Read the model definition and answer for the solid it produces. Units are mm, in the model's axes. A direction names the side the tool comes from. Round coordinates to 2 decimals unless told otherwise and drop trailing zeros. Order: outer loops, then holes, each group sorted by start corner. A loop starts at its lowest first (then second) coordinate and runs counter-clockwise, first axis right, second up. Notation, with made-up numbers: (-15.5, 70) - (-7.5, 70) arc R23 ccw to (-7.5, 86) - close; hole circle Ø9 at (-38, -32.5). An arc over 180 degrees is marked (long way). One line per question, with ' | ' between items. Start each with the question number.
1) For faces 1 (the flat face through (166, -2.794, 38)), 2 (the flat face through (-151, 2.794, -14)), 3 (the flat face through (-151, -2.794, -14)), determine the directions among +Z, -Z, +X, -X, +Y, -Y from which every point of the face is accessible in a straight line to the end or side of a thin tool.
2) The mould has two halves that part along X. Classify faces 4 (the flat face through (157.48, 6, 39)), 5 (the flat face through (166, 2.794, 38)), 6 (the cylindrical face through (-119.669, -0.133, -89.713)): pulls with the +X half, pulls with the -X half, needs draft (parallel to the pull), parting line crosses it, or undercut.
3) Flat-ended cylindrical pins translate along their axes: pin 1 (14 mm diameter, centred on x = -152, z = -16, fed in from -Y); pin 2 (2 mm diameter, centred on x = 55.88, y = 0, fed in from -Z); pin 3 (1 mm diameter, centred on y = 5.5, z = -12, fed in from +X). Find the tip coordinate at first contact, or state that the pin passes through.
4) The part is cut by section B-B, the plane z = -38.1. Give the vertices of the cut face in (x, y) (3 decimals), plus the area to 3 significant figures.
5) The part is cut by section C-C, the plane z = -77.5. Give the vertices of the cut face in (x, y) (3 decimals).
6) Straight lines are drawn through the part: line 1 (Z direction, x = -71.12, y = 2); line 2 (X direction, y = -0.5, z = 2.5); line 3 (X direction, y = 4.5, z = 66). For each, find the intervals that lie inside material, in ascending order. Write a range as from..to.
7) The part is cut by section A-A, the plane x = -118.11. Give the vertices of the cut face in (y, z) (3 decimals), plus the area to 3 significant figures.
8) The part is cut by section D-D, the plane x = 94. Give the vertices of the cut face in (y, z) (3 decimals).
from build123d import *

# Parameters (mm, degrees)
BOSS_EXTRUDE1_DEPTH       = 9.525
SKETCH2_W                 = 17.78
SKETCH2_H                 = 177.8
SKETCH2_H_2               = 76.2
BOSS_EXTRUDE2_DEPTH       = 2.794
F_1_4_CLEARANCE_HOLE1_D   = 6.7564
F_8_CLEARANCE_HOLE1_D     = 4.4958
F_1_4_CLEARANCE_HOLE2_D   = 6.7564
F_8_32_TAPPED_HOLE1_D     = 3.4544
F_8_32_TAPPED_HOLE1_DEPTH = 10.668
F_8_32_TAPPED_HOLE1_TIP   = 1.037806461
F_8_32_TAPPED_HOLE2_D     = 3.4544
F_8_32_TAPPED_HOLE2_DEPTH = 10.668
F_8_32_TAPPED_HOLE2_TIP   = 1.037806461


with BuildPart() as part:
    # Sketch1 → Boss-Extrude1 (new, symmetric)
    with BuildSketch(Plane(origin=(0, 0, 0), x_dir=(1, 0, 0), z_dir=(0, 1, 0))):
        with BuildLine():
            Line((0, 101.6), (-142.24, 101.6))
            Line((-142.24, 101.6), (-142.24, -76.2))
            Line((-142.24, -76.2), (-46.99, -76.2))
            ThreePointArc((-46.99, -76.2), (7.62, -51.017030863), (62.23, -76.2))
            Line((62.23, -76.2), (157.48, -76.2))
            Line((157.48, -76.2), (157.48, 0))
            Line((157.48, 0), (0, 0))
            Line((0, 0), (0, 101.6))
        make_face()
    extrude(amount=BOSS_EXTRUDE1_DEPTH, both=True)

    # Sketch2 → Boss-Extrude2 (add, symmetric)
    with BuildSketch(Plane(origin=(0, 0, 0), x_dir=(1, 0, 0), z_dir=(0, 1, 0))):
        with Locations((-151.13, 12.7)):
            Rectangle(SKETCH2_W, SKETCH2_H)
        with Locations((166.37, -38.1)):
            Rectangle(SKETCH2_W, SKETCH2_H_2)
    extrude(amount=BOSS_EXTRUDE2_DEPTH, both=True)

    # 1/4 Clearance Hole1 (through all)
    with Locations(Plane(origin=(0, 9.525, 0), x_dir=(1, 0, 0), z_dir=(0, 1, 0))):
        with Locations((-118.11, 92.71), (-118.11, 38.1), (-118.11, 0), (-118.11, -63.5)):
            Hole(F_1_4_CLEARANCE_HOLE1_D / 2)

    # #8 Clearance Hole1 (through all)
    with Locations(Plane(origin=(0, 9.525, 0), x_dir=(1, 0, 0), z_dir=(0, 1, 0))):
        with Locations((-101.6, 95.25), (-71.12, 95.25)):
            Hole(F_8_CLEARANCE_HOLE1_D / 2)

    # 1/4 Clearance Hole2 (through all)
    with Locations(Plane(origin=(0, 9.525, 0), x_dir=(1, 0, 0), z_dir=(0, 1, 0))):
        with Locations((146.05, -25.4), (146.05, -63.5)):
            Hole(F_1_4_CLEARANCE_HOLE2_D / 2)

    # #8-32 Tapped Hole1
    with Locations(Plane(origin=(0, 0, 0), x_dir=(-1, 0, 0), z_dir=(0, 0, -1))):
        with Locations((-137.16, 0), (-106.68, 0), (-55.88, 0), (-15.24, 0)):
            Hole(F_8_32_TAPPED_HOLE1_D / 2, depth=F_8_32_TAPPED_HOLE1_DEPTH)
            with Locations((0, 0, -(F_8_32_TAPPED_HOLE1_DEPTH + F_8_32_TAPPED_HOLE1_TIP / 2))):  # 118° drill point
                Cone(0, F_8_32_TAPPED_HOLE1_D / 2, F_8_32_TAPPED_HOLE1_TIP, mode=Mode.SUBTRACT)

    # #8-32 Tapped Hole2
    with Locations(Plane(origin=(0, 0, 0), x_dir=(0, 0, -1), z_dir=(1, 0, 0))):
        with Locations((69.85, 0), (25.4, 0)):
            Hole(F_8_32_TAPPED_HOLE2_D / 2, depth=F_8_32_TAPPED_HOLE2_DEPTH)
            with Locations((0, 0, -(F_8_32_TAPPED_HOLE2_DEPTH + F_8_32_TAPPED_HOLE2_TIP / 2))):  # 118° drill point
                Cone(0, F_8_32_TAPPED_HOLE2_D / 2, F_8_32_TAPPED_HOLE2_TIP, mode=Mode.SUBTRACT)


solid = part.part
Values:
1) face 1: +Z, -Z, +X, -Y | face 2: +Z, -Z, -X, +Y | face 3: +Z, -Z, -X, -Y
2) face 4: pulls with the +X half | face 5: needs draft | face 6: undercut
3) pin 1: stops at y = -2.79 | pin 2: stops at z = 11.1 | pin 3: stops at x = 0
4) outline: (-160.02, -2.794) - (-142.24, -2.794) - (-142.24, -9.525) - (-121.488, -9.525) - (-121.488, 9.525) - (-142.24, 9.525) - (-142.24, 2.794) - (-160.02, 2.794) - close; (-114.732, -9.525) - (0, -9.525) - (0, 9.525) - (-114.732, 9.525) - close | area: 2,680 mm^2
5) outline: (-160.02, -2.794) - (-142.24, -2.794) - (-142.24, -9.525) - (0, -9.525) - (0, 9.525) - (-142.24, 9.525) - (-142.24, 2.794) - (-160.02, 2.794) - close
6) line 1: z = -101.6..-97.5, -93..76.2 | line 2: x = -160.02..-120.38, -115.84..13.59, 16.89..54.23, 57.53..105.03, 108.33..135.51, 138.81..175.26 | line 3: x = -142.24..-120.38, -115.84..-36.28, 51.52..143.78, 148.32..157.48
7) outline: (-9.525, -101.6) - (9.525, -101.6) - (9.525, -96.088) - (-9.525, -96.088) - close; (-9.525, -89.332) - (9.525, -89.332) - (9.525, -41.478) - (-9.525, -41.478) - close; (-9.525, -34.722) - (9.525, -34.722) - (9.525, -3.378) - (-9.525, -3.378) - close; (-9.525, 3.378) - (9.525, 3.378) - (9.525, 60.122) - (-9.525, 60.122) - close; (-9.525, 66.878) - (9.525, 66.878) - (9.525, 76.2) - (-9.525, 76.2) - close | area: 2,870 mm^2
8) outline: (-9.525, 0) - (9.525, 0) - (9.525, 76.2) - (-9.525, 76.2) - close
